from build123d import *

# Parameters (mm, degrees)
EXTRUDE_1_DEPTH      = 3
EXTRUDE_2_DEPTH      = 2.5
EXTRUDE_2_DEPTH_BACK = 3.5
SKETCH_2_R           = 7.8
SKETCH_2_R_2         = 3.8
SKETCH_4_R           = 7.8
SKETCH_4_R_2         = 3.8
EXTRUDE_3_DEPTH      = 6
SKETCH_7_R           = 1.25
CUT_EXTRUDE_1_DEPTH  = 16


with BuildPart() as part:
    # Sketch 1 → Extrude 1 (new body)
    # profile 1 of 4: a face of its own
    with BuildSketch(Plane(origin=(0, 0, 0), x_dir=(1, 0, 0), z_dir=(0, 1, 0))):
        with BuildLine():
            Line((0, 4), (0, 6))
            Line((0, 6), (-15.5, 6))
            Line((-15.5, 6), (-15.5, -6))
            Line((-15.5, -6), (0, -6))
            Line((0, -6), (0, -4))
            Line((0, -4), (-2, -4))
            ThreePointArc((-2, -4), (-2.707106781, -3.707106781), (-3, -3))
            Line((-3, -3), (-3, 3))
            ThreePointArc((-3, 3), (-2.707106781, 3.707106781), (-2, 4))
            Line((-2, 4), (0, 4))
        make_face()
        with BuildLine():
            Line((-5.254817408, -0.9), (-13.615779121, -0.9))
            ThreePointArc((-13.615779121, -0.9), (-14.049888068, 0), (-13.615779121, 0.9))
            Line((-13.615779121, 0.9), (-5.254817408, 0.9))
            ThreePointArc((-5.254817408, 0.9), (-4.820708461, 0), (-5.254817408, -0.9))
        make_face(mode=Mode.SUBTRACT)
    # profile 2 of 4: a face of its own
    with BuildSketch(Plane(origin=(0, 0, 0), x_dir=(1, 0, 0), z_dir=(0, 1, 0))):
        Polygon((-15.5, -6), (-15.5, 6), (-18, 6), (-20.5, 6), (-20.5, -6), (-18, -6), align=None)
    # profile 3 of 4: a face of its own
    with BuildSketch(Plane(origin=(0, 0, 0), x_dir=(1, 0, 0), z_dir=(0, 1, 0))):
        with BuildLine():
            Line((15.5, -6), (15.5, 6))
            Line((15.5, 6), (0, 6))
            Line((0, 6), (0, 4))
            Line((0, 4), (2, 4))
            ThreePointArc((2, 4), (2.707106781, 3.707106781), (3, 3))
            Line((3, 3), (3, -3))
            ThreePointArc((3, -3), (2.707106781, -3.707106781), (2, -4))
            Line((2, -4), (0, -4))
            Line((0, -4), (0, -6))
            Line((0, -6), (15.5, -6))
        make_face()
        with BuildLine():
            Line((5.254817408, 0.9), (13.615779121, 0.9))
            ThreePointArc((13.615779121, 0.9), (14.049888068, 0), (13.615779121, -0.9))
            Line((13.615779121, -0.9), (5.254817408, -0.9))
            ThreePointArc((5.254817408, -0.9), (4.820708461, 0), (5.254817408, 0.9))
        make_face(mode=Mode.SUBTRACT)
    # profile 4 of 4: a face of its own
    with BuildSketch(Plane(origin=(0, 0, 0), x_dir=(1, 0, 0), z_dir=(0, 1, 0))):
        Polygon((18, 6), (15.5, 6), (15.5, -6), (18, -6), (20.5, -6), (20.5, 6), align=None)
    extrude(amount=EXTRUDE_1_DEPTH)

    # Sketch 2 → Extrude 2 (add, two sides: drawn at the far end of the back side and taken through both)
    with BuildSketch(Plane.ZY.offset(18).offset(-EXTRUDE_2_DEPTH_BACK)):
        with Locations((0, 8)):
            Circle(SKETCH_2_R)
        with Locations((0.029069435, 7.993834456)):
            Circle(SKETCH_2_R_2, mode=Mode.SUBTRACT)
    extrude(amount=EXTRUDE_2_DEPTH + EXTRUDE_2_DEPTH_BACK)

    # Sketch 4 → Extrude 3 (add)
    with BuildSketch(Plane(origin=(20.5, 0, 0), x_dir=(0, 0, -1), z_dir=(1, 0, 0))):
        with Locations((0, 8)):
            Circle(SKETCH_4_R)
        with Locations((0, 8)):
            Circle(SKETCH_4_R_2, mode=Mode.SUBTRACT)
    extrude(amount=-EXTRUDE_3_DEPTH)

    # Sketch 7 → Cut-Extrude 1 (cut)
    with BuildSketch(Plane(origin=(0, 7.993834456, 0), x_dir=(1, 0, 0), z_dir=(0, 1, 0))):
        with Locations(Location((-17.5, 0, 0), (0, 0, 90))):
            Circle(SKETCH_7_R)
        with Locations(Location((17.5, 0, 0), (0, 0, 90))):
            Circle(SKETCH_7_R)
    extrude(amount=CUT_EXTRUDE_1_DEPTH, mode=Mode.SUBTRACT)


solid = part.part
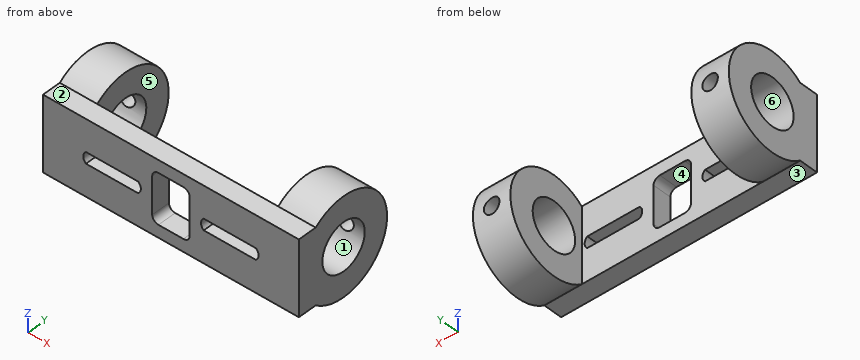
Geometry: final body of the model. Coordinates: model frame, mm. Face numbers are marked on the shaded views. A direction names the side the tool comes from. Coordinates: 2 decimals unless noted, no trailing zeros. Order: outer loops, then holes, each group sorted by start corner. A loop starts at its lowest first (then second) coordinate and runs counter-clockwise, first axis right, second up.
1) Section A-A (x = -7). Return loops of the section in (y, z), then the cut area to 3 significant figures.
Result sheet:
outline: (0, -6) - (3, -6) - (3, -0.9) - (0, -0.9) - close; (0, 0.9) - (3, 0.9) - (3, 6) - (0, 6) - close
area: 30.6 mm2
2) Section C-C (y = 14.75). Return loops of the section in (x, z).
Result sheet:
outline: (-20.5, -3.91) - (-14.5, -3.91) - (-14.5, 3.91) - (-20.5, 3.91) - close; (14.5, -3.91) - (20.5, -3.91) - (20.5, 3.91) - (14.5, 3.91) - close; hole circle Ø2.5 at (-17.5, 0); hole circle Ø2.5 at (17.5, 0)
3) Ray query, probe 1 along X at (y, z) = (14.4, 0); probe 2 along X at (y, z) = (4, -1.75); probe 3 along X at (y, z) = (15.25, -1). Return the intervals inside material, ascending.
Result sheet:
probe 1: x = -20.5 to -18.75, -16.25 to -14.5, 14.5 to 16.25, 18.75 to 20.5
probe 2: x = -20.5 to -14.5, 14.5 to 20.5
probe 3: x = -20.5 to -18.25, -16.75 to -14.5, 14.5 to 16.75, 18.25 to 20.5
4) Section B-B (y = 4.75). Return loops of the section in (x, z), then the cut area to 3 significant figures.
Result sheet:
outline: (-20.5, -7.09) - (-14.5, -7.09) - (-14.5, -1.95) - (-20.5, -1.95) - close; (-20.5, 2.01) - (-14.5, 2.01) - (-14.5, 7.09) - (-20.5, 7.09) - close; (14.5, -7.09) - (20.5, -7.09) - (20.5, -1.97) - (14.5, -1.97) - close; (14.5, 1.97) - (20.5, 1.97) - (20.5, 7.09) - (14.5, 7.09) - close
area: 123 mm2
5) First-contact query: P1, Ø2.5, axis at x = -10, y = 1, coming from the +Z side; P2, Ø1, axis at x = -16, z = 3.5, coming from the -Y side; P3, Ø6, axis at x = -7, y = 2.5, coming from the -Z side; P4, Ø1.5, axis at x = 5.5, z = -4, coming from the +Y side. Flat tips, straight axial feed; report the tip coordinate or a pass-through.
Result sheet:
P1: stops at z = 6
P2: stops at y = 0
P3: stops at z = -6
P4: stops at y = 3
6) Set-up query: the marked faces 4, 5 and 6. Return all of +Z, -Z, +X, -X, +Y, -Y with unobstructed straight access to the full face (end or side cutting, diameter ignored); none if empty.
Result sheet:
face 4: +Y, -Y
face 5: +Z, -Z, +Y
face 6: -X
7) Draft query along Z for the marked faces 1, 2 and 3. Return one class per face: released by +Z, released by -Z, zero draft, split by the parting line, or undercut.
Result sheet:
face 1: undercut
face 2: released by +Z
face 3: released by -Z
